Verification items for the finished model (mm, model axes). A direction names the side the tool comes from. Coordinates: 2 decimals unless noted, no trailing zeros. Order: outer loops, then holes, each group sorted by start corner. A loop starts at its lowest first (then second) coordinate and runs counter-clockwise, first axis right, second up. Notation, with made-up numbers: (36, 43) -> (40, 43) arc R22 ccw to (40, 72) -> close; hole circle Ø3 at (25.25, -9.5). An arc over 180 degrees is marked (long way). Answer as CSV lines item,"result".
Autodesk Inventor part; units mm, degrees
ref_plane "YZ Plane" through (0, 0, 0) normal (1, 0, 0) x (0, 1, 0)
ref_plane "XZ Plane" through (0, 0, 0) normal (0, 1, 0) x (-1, 0, 0)
ref_plane "XY Plane" through (0, 0, 0) normal (0, 0, 1) x (1, 0, 0)
sketch "Sketch1" plane through (0, 0, 0) normal (0, 1, 0) x (-1, 0, 0)
  line L0 (0, 0) -> (8, 0)
  line L1 (8, 0) -> (8, -50)
  line L2 (8, -50) -> (0, -50)
  line L3 (0, -50) -> (0, 0)
  dimension "d0" = 8
  dimension "d1" = 50
extrude "Extrusion1" add sketch "Sketch1" along normal blind 8
sketch "Sketch2" plane through (-8, 0, 0) normal (0, 0, 1) x (1, 0, 0)
  circle A0 centre (4, 4) radius 2.15
  point P0 (8, 0)
  dimension "d4" = 4.3
extrude "Extrusion2" cut sketch "Sketch2" against normal blind 4
sketch "Sketch3" plane through (0, 8, 0) normal (0, 1, 0) x (1, 0, 0)
  line L0 (-10.8104, 6) -> (3.7678, 6)
  line L1 (3.7678, 6) -> (3.7678, 4)
  line L2 (3.7678, 4) -> (-10.8104, 4)
  line L3 (-10.8104, 4) -> (-10.8104, 6)
  line L4 (-8, 0) -> (0, 0)
  dimension "d8" = 2
  dimension "d9" = 4
extrude "Extrusion3" cut sketch "Sketch3" against normal blind 6.2
sketch "Sketch4" plane through (-8, 8, -6) normal (0, 0, 1) x (1, 0, 0)
  circle A0 centre (4, -4) radius 2.15
  circle A1 centre (4, -4) radius 2.15
  point P0 (8, -8)
extrude "Extrusion4" cut sketch "Sketch4" against normal blind 40
sketch "Sketch5" plane through (0, 0, 0) normal (1, 0, 0) x (0, 0, -1)
  line L0 (6, 8) -> (50, 8)
  line L1 (6, 8) -> (10, 8)
  line L2 (10, 8) -> (15.6569, 2.3431)
  line L3 (15.6569, 2.3431) -> (40.6569, 2.3431)
  line L4 (6, 1.85) -> (46, 1.85)
  line L5 (40.6569, 2.3431) -> (46.3137, 8)
  line L6 (46.3137, 8) -> (10, 8)
  point P0 (0, 0)
  dimension "d14" = 4
  dimension "d15" = 8
  dimension "d16" = 135
  dimension "d17" = 25
  dimension "d18" = 135
extrude "Extrusion5" cut sketch "Sketch5" against normal blind 40
properties part number "ptfe_cutter_v6_40mm"
Item 1: Tool access check on faces 5 (the flat face through (-4, 8, -48)), 6 (the cylindrical face through (-3.01, 2.09, -1.97)), 7 (the flat face through (-3.944, 6.389, -44.703)). Record the directions out of +Z, -Z, +X, -X, +Y, -Y that give a thin tool (end or side, any length) a straight path to the whole face; none if there is none.
Answer list:
face 5,"+Z, -Z, +X, -X, +Y"
face 6,"+Z"
face 7,"+X, -X, +Y"
Item 2: Release check for a two-part mould opening along Z. For faces 1 (the flat face through (-3.9, 6.3, -4)), 2 (the flat face through (-1, 2.343, -28)), 3 (the flat face through (-4, 8, -8)), 4 (the flat face through (-4, 4, -50)) record: +Z half, -Z half, draft (parallel to the pull), parting line (faces both ways), or undercut.
Answer list:
face 1,"undercut"
face 2,"undercut"
face 3,"draft"
face 4,"-Z half"
Item 3: Section check B-B, the plane x = -4. Record the boundary of the cut face in (y, z), plus the area to 3 significant figures.
Answer list:
outline,"(0, -50) -> (8, -50) -> (8, -46.31) -> (6.15, -44.46) -> (6.15, -46) -> (1.85, -46) -> (1.85, -6) -> (1.8, -6) -> (1.8, -4) -> (1.85, -4) -> (1.85, 0) -> (0, 0) -> close; (6.15, -11.85) -> (8, -10) -> (8, -6) -> (6.15, -6) -> close; (6.15, -4) -> (8, -4) -> (8, 0) -> (6.15, 0) -> close"
area,"135 mm2"
Item 4: Section check A-A, the plane y = 5.25. Record the boundary of the cut face in (x, z).
Answer list:
outline,"(-8, -50) -> (0, -50) -> (0, -43.56) -> (-2.25, -43.56) -> (-2.25, -46) -> (-5.75, -46) -> (-5.75, -43.56) -> (-8, -43.56) -> close; (-8, -12.75) -> (-5.75, -12.75) -> (-5.75, -6) -> (-8, -6) -> close; (-8, -4) -> (-5.75, -4) -> (-5.75, 0) -> (-8, 0) -> close; (-2.25, -12.75) -> (0, -12.75) -> (0, -6) -> (-2.25, -6) -> close; (-2.25, -4) -> (0, -4) -> (0, 0) -> (-2.25, 0) -> close"
Item 5: Section check C-C, the plane z = -26. Record the boundary of the cut face in (x, y), plus the area to 3 significant figures.
Answer list:
outline,"(-8, 0) -> (0, 0) -> (0, 2.34) -> (-2.63, 2.34) arc R2.15 cw to (-5.37, 2.34) -> (-8, 2.34) -> close"
area,"17.8 mm2"
Item 6: Depth check by flat-ended pin: pin 1 Ø1.3 at (x, y) = (-3.5, 4) entering from +Z; pin 2 Ø1.3 at (x, z) = (-7.5, -31) entering from +Y; pin 3 Ø0.6 at (x, z) = (-3.5, -5.5) entering from +Y. Enter the tip coordinate at first touch or a pass-through.
Answer list:
pin 1,"z = -46"
pin 2,"y = 2.34"
pin 3,"y = 1.8"
Item 7: Section check D-D, the plane x = -6.75. Record the boundary of the cut face in (y, z).
Answer list:
outline,"(0, -50) -> (8, -50) -> (8, -46.31) -> (2.34, -40.66) -> (2.34, -15.66) -> (8, -10) -> (8, -6) -> (1.8, -6) -> (1.8, -4) -> (8, -4) -> (8, 0) -> (0, 0) -> close"
Item 8: Thickness scan on line 1 (Z direction, x = -3, y = 7.25); line 2 (Y direction, x = -4, z = -1.3); line 3 (Z direction, x = -1.75, y = 3.25). Record the ranges inside material, lowest first.
Answer list:
line 1,"-50 to -45.56, -10.75 to -6, -4 to 0"
line 2,"0 to 1.85, 6.15 to 8"
line 3,"-50 to -41.56, -14.75 to -6, -4 to 0"
